```python
from build123d import *

# Parameters (mm, degrees)
F0_W     = 580.39
F0_H     = 250.19
F1_DEPTH = 101.6
F2_T     = -12.7
F3_W     = 542.29
F3_H     = 184.15
F4_DEPTH = 25.4
F5_W     = 586.74
F5_H     = 215.9
F6_DEPTH = 12.7
F7_R     = 12.69999


# Not quite as in the source:
# - a fillet or chamfer is up to 0.001 mm smaller than in the source, because OpenCascade refuses the exact size


with BuildPart() as f1:
    # F0 (on Top) → F1 (new body, symmetric)
    with BuildSketch(Plane.XY):
        Rectangle(F0_W, F0_H)
    extrude(amount=F1_DEPTH, both=True)

    # F2
    f2_openings = [f1.faces().sort_by_distance(p)[0] for p in [
        (0, 0, 101.6),
    ]]
    offset(amount=F2_T, openings=f2_openings)

    # F3 (on face) → F4 (cut)
    with BuildSketch(Plane.XZ.offset(125.095)):
        with Locations((0, 9.525)):
            Rectangle(F3_W, F3_H)
    extrude(amount=-F4_DEPTH, mode=Mode.SUBTRACT)

    # F5 (on face) → F6 (join)
    with BuildSketch(Plane.XZ.offset(125.095)):
        Rectangle(F5_W, F5_H)
        Polygon((-290.195, -101.6), (-290.195, 101.6), (-271.145, 101.6), (-271.145, -82.55), (271.145, -82.55), (271.145, 101.6), (290.195, 101.6), (290.195, -101.6), align=None, mode=Mode.SUBTRACT)
        Polygon((-271.145, 101.6), (-290.195, 101.6), (-290.195, -101.6), (290.195, -101.6), (290.195, 101.6), (271.145, 101.6), (271.145, -82.55), (-271.145, -82.55), align=None)
    extrude(amount=F6_DEPTH)

    # F7 (radius 12.7 in the source; OpenCascade refuses exactly that, so slightly less here)
    f7_edges = [f1.edges().sort_by_distance(p)[0] for p in [
        (0, -137.795, 107.95),
        (-293.37, -137.795, 0),
        (0, -137.795, -107.95),
        (293.37, -137.795, 0),
    ]]
    fillet(f7_edges, radius=F7_R)


solid = f1.part
```
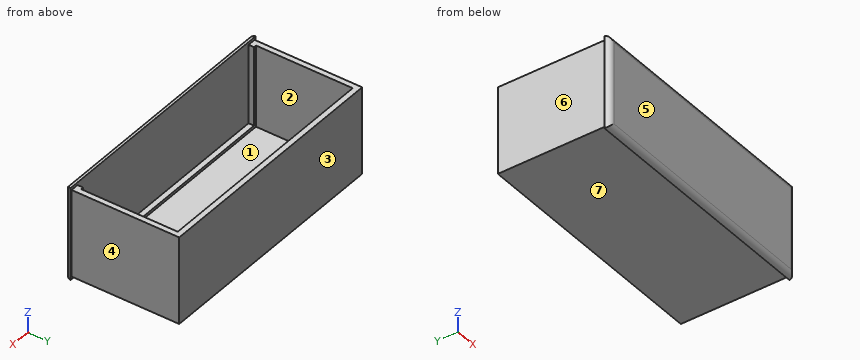
Part model, mm, in its own coordinate system. Face numbers are marked on the shaded views. A direction names the side the tool comes from. Give positions to 0.01 mm unless a question says otherwise; leave off trailing zeros. Write each loop counter-clockwise with the first axis right and the second up, starting at its lowest first coordinate (ties: lowest second). Pieces come first, ordered by that corner, then holes. Notation, with made-up numbers: (85.25, 32.25) -> (141.25, 32.25) arc R28 ccw to (141.25, 69.25) -> close; hole circle Ø8 at (-7, 51). An arc over 180 degrees is marked (long way). Put each result on its own line as item: value. Start each with the question number.
Item 1: Cut at C-C (y = 81.5). List the corners of the cut face in (x, z) (3 decimals), then the cut area to 3 significant figures.
Item 2: Pin check, flat tips, straight feed: pin 1 Ø10 at (x, y) = (-8.5, -55) entering from +Z; pin 2 Ø5 at (y, z) = (8.5, 84.5) entering from -X (3 decimals); pin 3 Ø10 at (y, z) = (9, -46) entering from +X (3 decimals). Stop position of each tip, or through.
Item 3: Which spindle directions (+Z, -Z, +X, -X, +Y, -Y) get a long thin tool onto all of the face, cutting with end or side? Do the marked faces 5, 6 and 7. Say none if no direction does.
Item 4: Pull direction Y, two halves, no side cores. Call the marked faces 1, 2, 3 and 4: pulls with the +Y half, pulls with the -Y half, needs draft (parallel to the pull), parting line crosses it, or undercut.
Item 5: Wall check: L1, parallel to X at y = -33.5, z = 4 (3 decimals); L2, parallel to Y at x = -138.5, z = -78 (3 decimals); L3, parallel to Z at x = -106.5, y = 93.5. Give the ranges that are in metal, low to high. Write a range as [from, to].
Answer list:
1. outline: (-290.195, -101.6) -> (290.195, -101.6) -> (290.195, 101.6) -> (277.495, 101.6) -> (277.495, -88.9) -> (-277.495, -88.9) -> (-277.495, 101.6) -> (-290.195, 101.6) -> close
1. area: 12,200 mm2
2. pin 1: stops at z = -88.9
2. pin 2: stops at x = -290.195
2. pin 3: stops at x = 290.195
3. face 5: +Z, -Z, +X, -X, -Y
3. face 6: +Z, -Z, -X, +Y
3. face 7: -Z, +X, -X, +Y
4. face 1: undercut
4. face 2: undercut
4. face 3: pulls with the +Y half
4. face 4: needs draft
5. L1: x = [-290.195, -277.495], [277.495, 290.195]
5. L2: y = [-137.795, -125.095], [112.395, 125.095]
5. L3: z = [-101.6, -88.9]
